Source: CAD feature listing. Evaluate the final solid. Frame: model axes, mm. A direction names the side the tool comes from. Coordinates: 2 decimals unless noted, no trailing zeros. Order: outer loops, then holes, each group sorted by start corner. A loop starts at its lowest first (then second) coordinate and runs counter-clockwise, first axis right, second up. Notation, with made-up numbers: (13.5, 19) - (65.5, 19) arc R20 ccw to (65.5, 30) - close; hole circle Ø1 at (73, -25). An arc over 180 degrees is marked (long way). One line per question, with ' | ' between items.
Autodesk Inventor part; units mm, degrees
ref_plane "YZ Plane" through (0, 0, 0) normal (1, 0, 0) x (0, 1, 0)
ref_plane "XZ Plane" through (0, 0, 0) normal (0, 1, 0) x (-1, 0, 0)
ref_plane "XY Plane" through (0, 0, 0) normal (0, 0, 1) x (1, 0, 0)
sketch "Sketch1" plane through (0, 0, 0) normal (0, 1, 0) x (-1, 0, 0)
  circle A0 centre (0, 0) radius 4
  dimension "d0" = 8
extrude "Extrusion1" add sketch "Sketch1" along normal blind 16.88
sketch "Sketch2" plane through (0, 16.88, 0) normal (0, 1, 0) x (1, 0, 0)
  point P0 (0, 0)
sketch "Sketch3" plane through (0, 0, 0) normal (0, -1, 0) x (1, 0, 0)
  point P0 (0, 0)
hole "Hole1" at (0, 0, 0) direction (0, 1, 0) diameter 3.78 depth 6 countersink diameter 4.5 countersink angle 90
hole "Hole2" at (0, 16.88, 0) direction (0, -1, 0) diameter 3.78 depth 6 countersink diameter 4.5 countersink angle 90
properties part number "Button Spacer"
(1) Cut plane B-B (y = 12.75). Return the cut outline in (x, z).
Taken from the geometry:
outline: circle Ø8 at (0, 0); hole circle Ø3.78 at (0, 0)
(2) Pin query (flat end, axial travel): P1, Ø3, axis at x = 0, z = 0, coming from the +Y side; P2, Ø3.5, axis at x = 0, z = 0, coming from the -Y side. Return the tip coordinate at first contact, or that it passes through.
Taken from the geometry:
P1: stops at y = 10.88 | P2: stops at y = 6
(3) Set-up query: faces 1 (the flat face through (0, 6, 0)), 2 (the flat face through (-2, 0, -2)), 3 (the cylindrical face through (1.845, 13.661, -0.41)). Return all of +Z, -Z, +X, -X, +Y, -Y with unobstructed straight access to the full face (end or side cutting, diameter ignored); none if empty.
Taken from the geometry:
face 1: -Y | face 2: +Z, -Z, +X, -X, -Y | face 3: +Y
(4) Cut plane A-A (x = 0). Return the cut outline in (y, z), and give its area (3 significant figures).
Taken from the geometry:
outline: (0, -4) - (16.88, -4) - (16.88, -2.25) - (16.52, -1.89) - (10.88, -1.89) - (10.88, 1.89) - (16.52, 1.89) - (16.88, 2.25) - (16.88, 4) - (0, 4) - (0, 2.25) - (0.36, 1.89) - (6, 1.89) - (6, -1.89) - (0.36, -1.89) - (0, -2.25) - close | area: 89.4 mm²
(5) Cut plane D-D (y = 6.5). Return the cut outline in (x, z).
Taken from the geometry:
outline: circle Ø8 at (0, 0)
(6) Material intervals for L1, parallel to Z at x = 0, y = 1.5; L2, parallel to Y at x = -1.25, z = 1; L3, parallel to Z at x = 1, y = 14.75, sorted ascending. Write a range as from..to.
Taken from the geometry:
L1: z = -4..-1.89, 1.89..4 | L2: y = 6..10.88 | L3: z = -3.87..-1.6, 1.6..3.87
(7) Pull-direction query (Z, two-part tool) for faces 4 (the cylindrical face through (0.867, 8.322, 3.905)), 5 (the flat face through (-2, 16.88, -2)), 6 (the flat face through (0, 10.88, 0)); classes: pulls with the +Z half, pulls with the -Z half, needs draft (parallel to the pull), parting line crosses it, or undercut.
Taken from the geometry:
face 4: parting line crosses it | face 5: needs draft | face 6: undercut
(8) Cut plane C-C (z = 0). Return the cut outline in (x, y), and give its area (3 significant figures).
Taken from the geometry:
outline: (-4, 0) - (-2.25, 0) - (-1.89, 0.36) - (-1.89, 6) - (1.89, 6) - (1.89, 0.36) - (2.25, 0) - (4, 0) - (4, 16.88) - (2.25, 16.88) - (1.89, 16.52) - (1.89, 10.88) - (-1.89, 10.88) - (-1.89, 16.52) - (-2.25, 16.88) - (-4, 16.88) - close | area: 89.4 mm²
